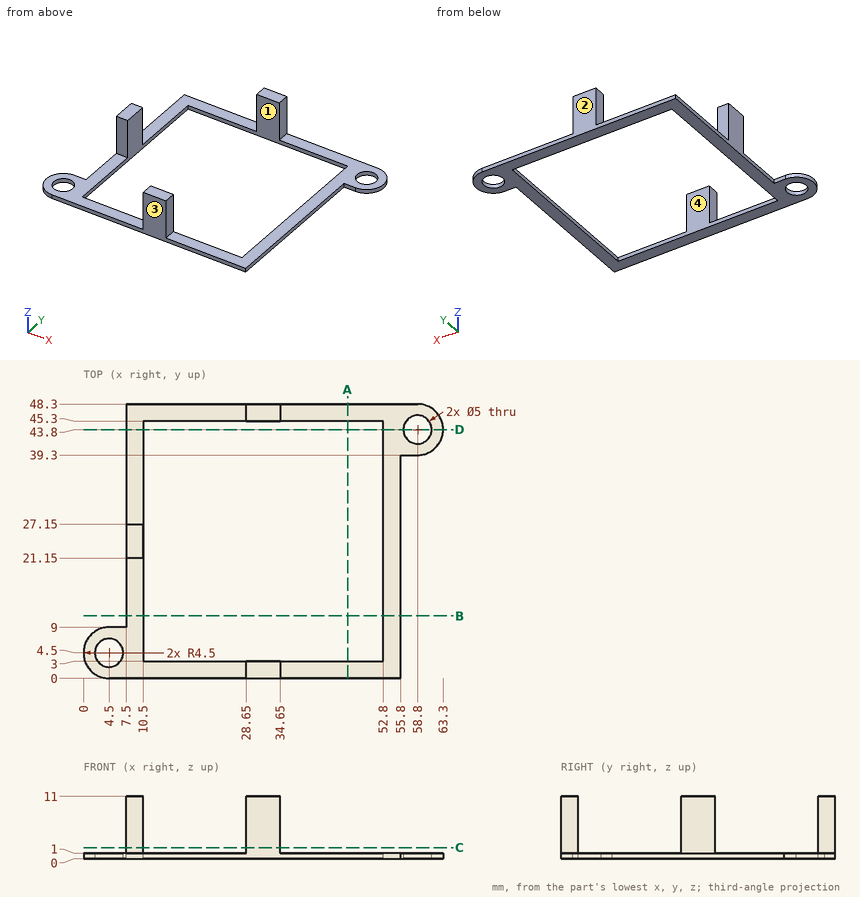
Print and shaded views of the part. All mm, measured from the part's lowest x, y and z. Give positions to 0.01 mm unless a question says otherwise; leave off trailing zeros. Loops run counter-clockwise (first coordinate to the right, second up) from the corner with the lowest first, then second, coordinate; pieces in that order, holes last. Notation, with made-up numbers: M -28.75,-22 L 13.25,-22 A23 ccw 13.25,13 Z; hole C 68.25,51 d3. An arc over 180 degrees is marked long. Write each question's results on one line, items separated by ' | '.
Q1. Band-saw the part on D-D on y = 43.8. Write the cut outline in (x, z).
Geometry check:
outline: M 7.5,0 L 10.5,0 L 10.5,1 L 7.5,1 Z; M 52.8,0 L 56.3,0 L 56.3,1 L 52.8,1 Z; M 61.3,0 L 63.3,0 L 63.3,1 L 61.3,1 Z
Q2. Band-saw the part on A-A on x = 46.5. Write the cut outline in (y, z), and give its area (3 significant figures).
Geometry check:
outline: M 0,0 L 3,0 L 3,1 L 0,1 Z; M 45.3,0 L 48.3,0 L 48.3,1 L 45.3,1 Z | area: 6.00 mm²
Q3. Band-saw the part on C-C on z = 2. Write the cut outline in (x, y), and give its area (3 significant figures).
Geometry check:
outline: M 7.5,21.15 L 10.5,21.15 L 10.5,27.15 L 7.5,27.15 Z; M 28.65,0 L 34.65,0 L 34.65,3 L 28.65,3 Z; M 28.65,45.3 L 34.65,45.3 L 34.65,48.3 L 28.65,48.3 Z | area: 54.0 mm²
Q4. Probe probe 1 along Y at (x, z) = (4.5, 0.7); probe 2 along Y at (x, z) = (9, 4); probe 3 along X at (y, z) = (22.5, 2.75). List the from-to ranges inside material, lowest first.
Geometry check:
probe 1: y = 0 to 2, 7 to 9 | probe 2: y = 21.15 to 27.15 | probe 3: x = 7.5 to 10.5
Q5. Band-saw the part on B-B on y = 11. Write the cut outline in (x, z), and give its area (3 significant figures).
Geometry check:
outline: M 7.5,0 L 10.5,0 L 10.5,1 L 7.5,1 Z; M 52.8,0 L 55.8,0 L 55.8,1 L 52.8,1 Z | area: 6.00 mm²
Q6. Flat gauge pins, fed straight in: P1, Ø6, axis at x = 46.5, z = 6.5, coming from the -Y side; P2, Ø5, axis at x = 25.5, z = 1.5, coming from the +Y side; P3, Ø1, axis at x = 10.5, z = 2, coming from the +Y side; P4, Ø6.5, axis at x = 12, y = 12, coming from the +Z side. Where does each tip first touch, or does it go through?
Geometry check:
P1: passes through | P2: stops at y = 48.3 | P3: stops at y = 27.15 | P4: stops at z = 1
Q7. Mould opens along Y. For the marked faces 1, 2, 3 and 4 say: pulls with the +Y half, pulls with the -Y half, needs draft (parallel to the pull), parting line crosses it, or undercut.
Geometry check:
face 1: undercut | face 2: pulls with the +Y half | face 3: pulls with the -Y half | face 4: undercut
